Autodesk Inventor part; units mm, degrees
ref_plane "YZ Plane" through (0, 0, 0) normal (1, 0, 0) x (0, 1, 0)
ref_plane "XZ Plane" through (0, 0, 0) normal (0, 1, 0) x (-1, 0, 0)
ref_plane "XY Plane" through (0, 0, 0) normal (0, 0, 1) x (1, 0, 0)
sketch "Sketch1" plane through (0, 0, 0) normal (0, 0, 1) x (1, 0, 0)
  line L0 (0, 0) -> (19, 0)
  line L1 (19, 0) -> (19, 2000)
  line L2 (19, 2000) -> (0, 2000)
  line L3 (0, 2000) -> (0, 0)
  dimension "d0" = 19
  dimension "d1" = 2000
extrude "Extrusion1" add sketch "Sketch1" along normal blind 10
sketch "Sketch2" plane through (0, 0, 10) normal (0, 0, 1) x (1, 0, 0)
  line L0 (19, 0) -> (19, 2000)
  line L1 (19, 2000) -> (0, 2000)
  line L2 (0, 2000) -> (0, 0)
  line L3 (0, 0) -> (19, 0)
  line L4 (0, 2000) -> (19, 1981)
  dimension "d7" = 45
extrude "Extrusion2" cut sketch "Sketch2" against normal blind 10 contours L4 L1 L0
sketch "Sketch3" plane through (0, 0, 10) normal (0, 0, 1) x (1, 0, 0)
  circle A0 centre (9.5, 210) radius 3
  circle A1 centre (9.5, 170) radius 3
  line L0 (0, 0) -> (19, 0)
  point P0 (9.5, 0)
  dimension "d8" = 6
  dimension "d9" = 40
  dimension "d10" = 170
extrude "Extrusion3" cut sketch "Sketch3" against normal blind 10
sketch "Sketch4" plane through (0, 0, 10) normal (0, 0, 1) x (1, 0, 0)
  circle A0 centre (9.5, 1815) radius 3
  line L0 (19, 1981) -> (0, 2000)
  circle A1 centre (9.5, 1775) radius 3
  point P0 (0, 0)
  point P1 (9.5, 1990.5)
  dimension "d14" = 185
  dimension "d15" = 6
  dimension "d16" = 40
extrude "Extrusion4" cut sketch "Sketch4" against normal blind 10
properties part number "Dichtung_links"
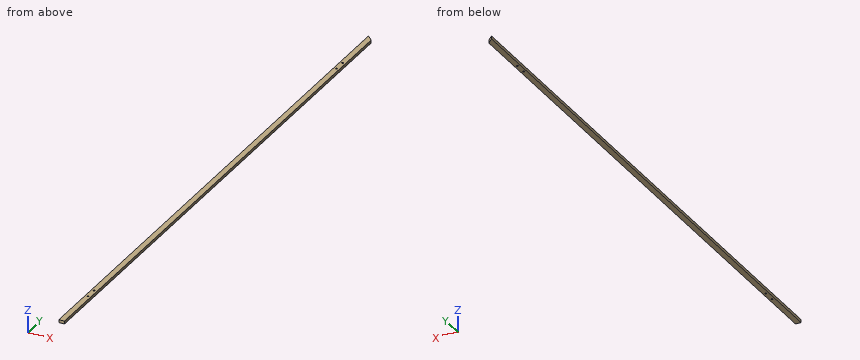
Design review of the part built by this model. Coordinates are the model's own, in mm. Give positions to 0.01 mm unless a question says otherwise; leave off trailing zeros. Write each loop counter-clockwise with the first axis right and the second up, starting at its lowest first coordinate (ties: lowest second). Pieces come first, ordered by that corner, then holes. Notation, with made-up numbers: M 45,56.25 L 86,56.25 A17 ccw 86,69.25 Z; hole C 6.25,15 d7. An arc over 180 degrees is marked long. Return JSON: item names as keys, results as strings. Group by question number.
Item 1: Clearance check with a flat-ended pin moving along its axis: pin 1 Ø3.5 at (x, y) = (9.5, 1775) entering from +Z. State where the tip first meets the part, or that it passes through.
Item 2: Take a section at A-A (x = 9.5). Give the boundary of the cut face in (y, z).
Item 3: Wall thickness on line 1 along X through (y, z) = (1815, 2.75); line 2 along Y through (x, z) = (9.5, 2.5); line 3 along Y through (x, z) = (9, 5): over which ranges is each line inside the solid? List them lowest first.
Return value:
{
 "1": {"pin 1": "passes through"},
 "2": {"outline": "M 0,0 L 167,0 L 167,10 L 0,10 Z; M 173,0 L 207,0 L 207,10 L 173,10 Z; M 213,0 L 1772,0 L 1772,10 L 213,10 Z; M 1778,0 L 1812,0 L 1812,10 L 1778,10 Z; M 1818,0 L 1990.5,0 L 1990.5,10 L 1818,10 Z"},
 "3": {"line 1": "x = 0 to 6.5, 12.5 to 19", "line 2": "y = 0 to 167, 173 to 207, 213 to 1772, 1778 to 1812, 1818 to 1990.5", "line 3": "y = 0 to 167.04, 172.96 to 207.04, 212.96 to 1772.04, 1777.96 to 1812.04, 1817.96 to 1991"}
}
